For this review, take the finished solid that the model builds, in its own axes (mm). A direction names the side the tool comes from. Round coordinates to 2 decimals unless told otherwise and drop trailing zeros. Write each loop counter-clockwise with the first axis right and the second up, starting at its lowest first coordinate (ties: lowest second). Pieces come first, ordered by that corner, then holes. Notation, with made-up numbers: M 30,53.5 L 58,53.5 A21 cw 58,63.5 Z; hole C -24.75,42.25 d6. An arc over 180 degrees is marked long. Use one line per item in the form item = value. Start each with the question number.
Item 1: Add section A-A (y = -76.01). State the section outline as (x, z) points, and give its area (3 significant figures).
Item 2: Draft analysis for pull direction Y (two halves, no side actions). For faces 6 (the cylindrical face through (13.284, 2.265, 1.521)), 7 (the flat face through (19, -82, 0)), 8 (the flat face through (29.44, -154.176, 1.479)), state which applies: released by +Y, released by -Y, zero draft, split by the parting line, or undercut.
Item 3: For P1, Ø1, axis at x = 15, z = 2, coming from the +Y side; P2, Ø0.9, axis at y = -84.5, z = 2, coming from the -X side; P3, Ø0.9, axis at y = -31, z = 2, coming from the +X side, all flat-tipped, find the tip position at first contact; note any pin that passes through.
Item 4: Add section B-B (x = 0). State the section outline as (y, z) points, and give its area (3 significant figures).
Item 5: Add section D-D (y = -46). State the section outline as (x, z) points, and give its area (3 significant figures).
Item 6: Add section C-C (x = 41). State the section outline as (y, z) points.
Item 7: For faces 1 (the flat face through (38.54, -71.87, 1.52)), 2 (the flat face through (4, -162, 1)), 3 (the cylindrical face through (14.603, -144.162, 1.479)), 4 (the flat face through (19, -82, 3)), 5 (the flat face through (-1, -17, 1)), list the 3-axis set-ups (+Z, -Z, +X, -X, +Y, -Y) from which the entire face can be reached by the end or side of a thin tool; tool diameter is ignored.
Item 8: For line 1 (Y direction, x = 0, z = 0.8); line 2 (X direction, y = -165.02, z = 1.35); line 3 (X direction, y = -139.02, z = 1.75), list the stretches that pass through material, from the lowest coordinate up. Write a range as [from, to].
from build123d import *

# Parameters (mm, degrees)
SKETCH_1_R      = 1.55
EXTRUDE_1_DEPTH = 3
FILLET_1_R      = 2
SKETCH_2_R      = 1.6
EXTRUDE_2_DEPTH = 3
FILLET_2_R      = 10
SKETCH_4_R      = 1.6
EXTRUDE_3_DEPTH = 3
FILLET_3_R      = 10


with BuildPart() as part:
    # 草图1 → 凸台-拉伸1 (new body)
    with BuildSketch(Plane.XY):
        with BuildLine():
            Line((4, -17), (-4, -17))
            Line((-4, -17), (-4, 17))
            Line((-4, 17), (4, 17))
            Line((4, 17), (4, 3))
            ThreePointArc((4, 3), (18.142135624, -2.857864376), (24, -17))
            Line((24, -17), (24, -135.02))
            ThreePointArc((24, -135.02), (18.142135624, -149.162135624), (4, -155.02))
            Line((4, -155.02), (4, -169.02))
            Line((4, -169.02), (-4, -169.02))
            Line((-4, -169.02), (-4, -135.02))
            Line((-4, -135.02), (4, -135.02))
            Line((4, -135.02), (4, -149.02))
            ThreePointArc((4, -149.02), (13.899494937, -144.919494937), (18, -135.02))
            Line((18, -135.02), (18, -17))
            ThreePointArc((18, -17), (13.899494937, -7.100505063), (4, -3))
            Line((4, -3), (4, -17))
        make_face()
        with Locations((0, 13)):
            Circle(SKETCH_1_R, mode=Mode.SUBTRACT)
        with Locations((0, -13)):
            Circle(SKETCH_1_R, mode=Mode.SUBTRACT)
        with Locations((0, -139.02)):
            Circle(SKETCH_1_R, mode=Mode.SUBTRACT)
        with Locations((0, -165.02)):
            Circle(SKETCH_1_R, mode=Mode.SUBTRACT)
    extrude(amount=EXTRUDE_1_DEPTH)

    # 圆角1
    fillet_1_edges = [part.edges().sort_by_distance(p)[0] for p in [
        (4, -3, 1.5),
        (4, -17, 1.5),
        (4, 17, 1.5),
        (4, 3, 1.5),
        (4, -155.02, 1.5),
        (4, -169.02, 1.5),
        (4, -135.02, 1.5),
        (4, -149.02, 1.5),
    ]]
    fillet(fillet_1_edges, radius=FILLET_1_R)

    # 草图2 → 凸台-拉伸2 (add)
    with BuildSketch(Plane.XY):
        with BuildLine():
            Line((13.058826075, 0.830806772), (28.763705104, 12.66528197))
            ThreePointArc((28.763705104, 12.66528197), (33.344931419, 12.344931419), (33.66528197, 7.763705104))
            Line((33.66528197, 7.763705104), (21.830806772, -7.941173925))
            ThreePointArc((21.830806772, -7.941173925), (18.142135624, -2.857864376), (13.058826075, 0.830806772))
        make_face()
        with Locations((30.870057685, 9.870057685)):
            Circle(SKETCH_2_R, mode=Mode.SUBTRACT)
    extrude_2 = extrude(amount=EXTRUDE_2_DEPTH)

    # 镜向5: 凸台-拉伸2 across plane
    add(extrude_2.mirror(Plane.ZX.offset(-76.01)))

    # 圆角2
    fillet_2_edges = [part.edges().sort_by_distance(p)[0] for p in [
        (21.830806772, -7.941173925, 1.5),
        (13.058826075, 0.830806772, 1.5),
        (21.830806772, -144.078826075, 1.5),
        (13.058826075, -152.850806772, 1.5),
    ]]
    fillet(fillet_2_edges, radius=FILLET_2_R)

    # 草图4 → 凸台-拉伸3 (add)
    with BuildSketch(Plane.XY.offset(3)):
        Polygon((24, -69.307133405), (45, -73.01), (45, -79.01), (24, -82.712866595), align=None)
        with Locations((41, -76.01)):
            Circle(SKETCH_4_R, mode=Mode.SUBTRACT)
    extrude(amount=-EXTRUDE_3_DEPTH)

    # 圆角3
    fillet_3_edges = [part.edges().sort_by_distance(p)[0] for p in [
        (24, -69.307133405, 1.5),
        (24, -82.712866595, 1.5),
    ]]
    fillet(fillet_3_edges, radius=FILLET_3_R)


solid = part.part
Calculated:
q1.outline = M 18,0 L 39.4,0 L 39.4,3 L 18,3 Z; M 42.6,0 L 45,0 L 45,3 L 42.6,3 Z
q1.area = 71.4 mm^2
q2.face_6 = released by +Y
q2.face_7 = zero draft
q2.face_8 = undercut
q3.P1 = 2.97
q3.P2 = 18
q3.P3 = 24
q4.outline = M -169.02,0 L -166.57,0 L -166.57,3 L -169.02,3 Z; M -163.47,0 L -140.57,0 L -140.57,3 L -163.47,3 Z; M -137.47,0 L -135.02,0 L -135.02,3 L -137.47,3 Z; M -17,0 L -14.55,0 L -14.55,3 L -17,3 Z; M -11.45,0 L 11.45,0 L 11.45,3 L -11.45,3 Z; M 14.55,0 L 17,0 L 17,3 L 14.55,3 Z
q4.area = 167 mm^2
q5.outline = M 18,0 L 24,0 L 24,3 L 18,3 Z
q5.area = 18.0 mm^2
q6.outline = M -79.72,0 L -77.61,0 L -77.61,3 L -79.72,3 Z; M -74.41,0 L -72.3,0 L -72.3,3 L -74.41,3 Z
q7.face_1 = +Z, -Z, +X
q7.face_2 = +Z, -Z, -Y
q7.face_3 = +Z, -Z
q7.face_4 = +Z, +X, -X, +Y, -Y
q7.face_5 = +Z, -Z, -X
q8.line_1 = [-169.02, -166.57], [-163.47, -140.57], [-137.47, -135.02], [-17, -14.55], [-11.45, 11.45], [14.55, 17]
q8.line_2 = [-4, -1.55], [1.55, 4], [29.3, 32.44]
q8.line_3 = [-4, -1.55], [1.55, 4], [17.42, 23.6]
